```python
from build123d import *

# Parameters (mm, degrees)
SKETCH1_R               = 20
BOSS_EXTRUDE1_DEPTH     = 130
BOSS_EXTRUDE2_DEPTH     = 5
SKETCH3_R               = 5
BOSS_EXTRUDE3_DEPTH     = 10
SKETCH4_W               = 11.5
SKETCH4_H               = 30
BOSS_EXTRUDE4_DEPTH     = 20
FILLET1_R               = 10
CUT_EXTRUDE1_DEPTH      = 154.502646557
CUT_EXTRUDE1_DEPTH_BACK = 154.502646557
SKETCH5_R               = 5


with BuildPart() as part:
    # Sketch1 → Boss-Extrude1 (new body)
    with BuildSketch(Plane.XY):
        Circle(SKETCH1_R)
    extrude(amount=BOSS_EXTRUDE1_DEPTH)

    # Sketch2 → Boss-Extrude2 (add, symmetric)
    with BuildSketch(Plane(origin=(0, 0, 0), x_dir=(1, 0, 0), z_dir=(0, 1, 0))):
        Polygon((23, -72.5), (15.5, -65), (23, -57.5), (8, -57.5), (8, -72.5), align=None)
    extrude(amount=BOSS_EXTRUDE2_DEPTH, both=True)

    # Sketch3 → Boss-Extrude3 (add)
    with BuildSketch(Plane(origin=(0, 0, 0), x_dir=(-1, 0, 0), z_dir=(0, 0, -1))):
        with Locations(Location((0, 0, 0), (0, 0, 180))):
            Circle(SKETCH3_R)
    extrude(amount=BOSS_EXTRUDE3_DEPTH)

    # Sketch4 → Boss-Extrude4 (add)
    with BuildSketch(Plane.XY.offset(130)):
        Rectangle(SKETCH4_W, SKETCH4_H)
    extrude(amount=BOSS_EXTRUDE4_DEPTH)

    # Fillet1
    fillet1_edges = [part.edges().sort_by_distance(p)[0] for p in [
        (0, -15, 150),
        (0, 15, 150),
    ]]
    fillet(fillet1_edges, radius=FILLET1_R)

    # Sketch5 → Cut-Extrude1 (cut, two sides: drawn at the far end of the back side and taken through both)
    with BuildSketch(Plane(origin=(5.75, 0, 0), x_dir=(0, 0, -1), z_dir=(1, 0, 0)).offset(-CUT_EXTRUDE1_DEPTH_BACK)):
        with Locations(Location((-140, 0, 0), (0, 0, 90))):
            Circle(SKETCH5_R)
    extrude(amount=CUT_EXTRUDE1_DEPTH + CUT_EXTRUDE1_DEPTH_BACK, mode=Mode.SUBTRACT)


solid = part.part
```
Input: part model. Units: mm. Frame: model coordinates. A direction names the side the tool comes from. Coordinates: 2 decimals unless noted, no trailing zeros. Loops run counter-clockwise (first coordinate to the right, second up) from the corner with the lowest first, then second, coordinate; pieces in that order, holes last.
Q1. Contact query for flat-ended pins moving along their axis: pin 1 (10 mm diameter, centred on x = -14, y = 6.5, fed in from -Z); pin 2 (4 mm diameter, centred on x = 21, y = -0.5, fed in from +Z); pin 3 (1.8 mm diameter, centred on x = 21.5, z = 70, fed in from -Y); pin 4 (6 mm diameter, centred on y = 0, z = 140, fed in from -X). Output: stop coordinate, or through.
Results are:
pin 1: stops at z = 0
pin 2: stops at z = 130
pin 3: stops at y = -5
pin 4: passes through
Q2. Mould query, pull axis Y, two halves, no side actions, for faces 1 (the cylindrical face through (0.08, 12.15, 146.99)), 2 (the cylindrical face through (-0.081, 2.307, 135.564)), 3 (the flat face through (9, 0, 130)). Classes: +Y half, -Y half, draft (parallel to the pull), parting line (faces both ways), or undercut.
Results are:
face 1: +Y half
face 2: undercut
face 3: draft
Q3. Section D-D, the plane y = 9.5. Return the cut outline in (x, z), and give its area (3 significant figures).
Results are:
outline: (-17.6, 0) - (17.6, 0) - (17.6, 130) - (5.75, 130) - (5.75, 148.93) - (-5.75, 148.93) - (-5.75, 130) - (-17.6, 130) - close
area: 4,790 mm2
Q4. Section C-C, the plane z = 137. Return the cut outline in (x, y).
Results are:
outline: (-5.75, -15) - (5.75, -15) - (5.75, -4) - (-5.75, -4) - close; (-5.75, 4) - (5.75, 4) - (5.75, 15) - (-5.75, 15) - close
Q5. Line query: line 1 along Y through (x, z) = (2.5, 140); line 2 along Z through (x, y) = (-1, 0); line 3 along Z through (x, y) = (0, -1.5). Output: solid intervals per line, ascending.
Results are:
line 1: y = -15 to -5, 5 to 15
line 2: z = -10 to 135, 145 to 150
line 3: z = -10 to 135.23, 144.77 to 150
Q6. Section B-B, the plane y = 2. Return the cut outline in (x, z).
Results are:
outline: (-19.9, 0) - (-4.58, 0) - (-4.58, -10) - (4.58, -10) - (4.58, 0) - (19.9, 0) - (19.9, 57.5) - (23, 57.5) - (19.9, 60.6) - (19.9, 69.4) - (23, 72.5) - (19.9, 72.5) - (19.9, 130) - (5.75, 130) - (5.75, 135.42) - (-5.75, 135.42) - (-5.75, 130) - (-19.9, 130) - close; (-5.75, 144.58) - (5.75, 144.58) - (5.75, 150) - (-5.75, 150) - close
Q7. Set-up query: faces 4 (the flat face through (20, -5, 71)), 5 (the flat face through (-5.75, 3, 135)), 6 (the cylindrical face through (-5, 0, -5)), 7 (the flat face through (0, 15, 135)), 8 (the flat face through (21, 5, 59)). Return all of +Z, -Z, +X, -X, +Y, -Y with unobstructed straight access to the full face (end or side cutting, diameter ignored); none if empty.
Results are:
face 4: +Z, -Z, +X, -Y
face 5: +Z, -X, +Y, -Y
face 6: -Z
face 7: +Z, +X, -X, +Y
face 8: +Z, -Z, +X, +Y
Q8. Section A-A, the plane x = 0. Return the cut outline in (y, z), and give its area (3 significant figures).
Results are:
outline: (-20, 0) - (-5, 0) - (-5, -10) - (5, -10) - (5, 0) - (20, 0) - (20, 130) - (15, 130) - (15, 140) arc R10 ccw to (5, 150) - (-5, 150) arc R10 ccw to (-15, 140) - (-15, 130) - (-20, 130) - close; hole circle Ø10 at (0, 140)
area: 5,780 mm2
